Here's the drawing with two shaded views (mm, measured from the low corner). I have some questions. A direction names the side the tool comes from. Round coordinates to 2 decimals unless told otherwise and drop trailing zeros. Loops run counter-clockwise (first coordinate to the right, second up) from the corner with the lowest first, then second, coordinate; pieces in that order, holes last. Notation, with made-up numbers: (46, 34) -> (91, 34) arc R20 ccw to (91, 68) -> close; hole circle Ø11 at (58.25, 61.25). An arc over 180 degrees is marked (long way). Write each question's results on one line, items separated by ' | '.
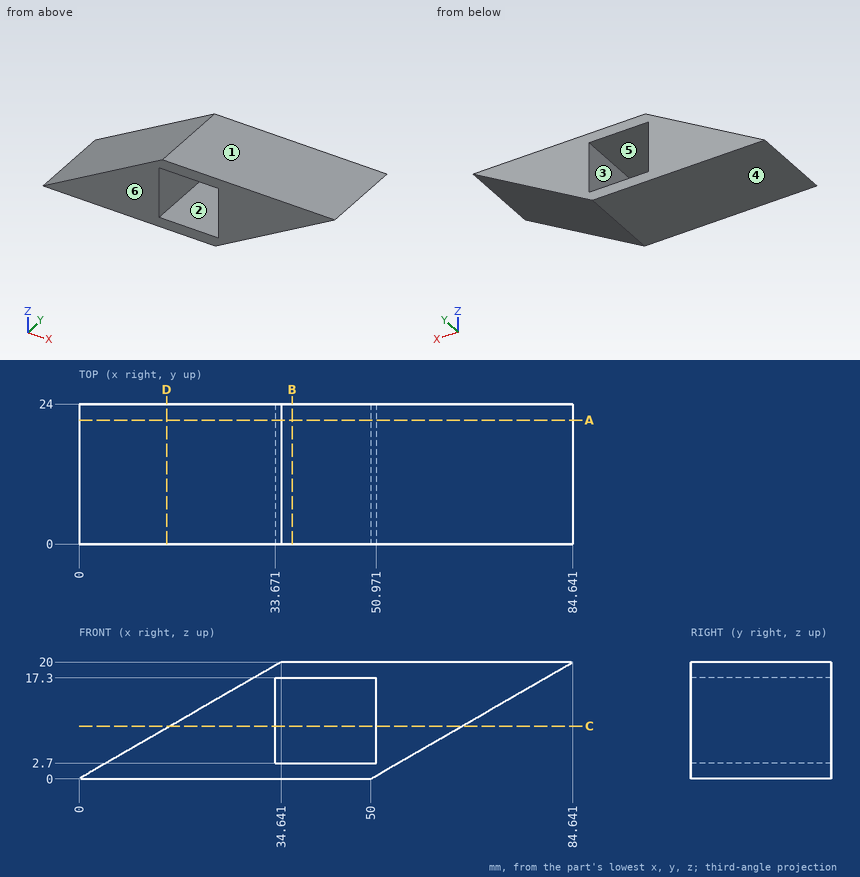
1. Will these pins go through, and if not, where does the flat tip stop? pin 1 (6 mm diameter, centred on y = 11.5, z = 5.5, fed in from +X) (1 decimal); pin 2 (5 mm diameter, centred on x = 25, y = 17, fed in from +Z); pin 3 (11.5 mm diameter, centred on y = 13, z = 12.5, fed in from -X).
Final values:
pin 1: x = 64.7 | pin 2: z = 15.88 | pin 3: x = 11.69
2. Please list where these lines run through material, in increasing order: line 1 (Z direction, x = 44.5, y = 16.25); line 2 (X direction, y = 20, z = 13.25); line 3 (X direction, y = 3, z = 3.75) (1 decimal). Write a range as from..to.
Final values:
line 1: 0..2.7, 17.3..20 | line 2: 22.95..33.67, 50.97..72.95 | line 3: 6.5..33.7, 51..56.5
3. We'd pull the mould along Z, two halves only. Please class the marked faces 3, 4, 5 and 6: pulls with the +Z half, pulls with the -Z half, needs draft (parallel to the pull), parting line crosses it, or undercut.
Final values:
face 3: undercut | face 4: pulls with the -Z half | face 5: undercut | face 6: needs draft
4. If we section it at A-A (y = 21.25): List the corners of the cut face in (x, z) for me.
Final values:
outline: (0, 0) -> (50, 0) -> (84.64, 20) -> (34.64, 20) -> close; hole (33.67, 2.7) -> (50.97, 2.7) -> (50.97, 17.3) -> (33.67, 17.3) -> close
5. If we section it at B-B (x = 36.5): List the corners of the cut face in (y, z) for me.
Final values:
outline: (0, 0) -> (24, 0) -> (24, 2.7) -> (0, 2.7) -> close; (0, 17.3) -> (24, 17.3) -> (24, 20) -> (0, 20) -> close
6. If we section it at C-C (z = 9): List the corners of the cut face in (x, y) for me.
Final values:
outline: (15.59, 0) -> (33.67, 0) -> (33.67, 24) -> (15.59, 24) -> close; (50.97, 0) -> (65.59, 0) -> (65.59, 24) -> (50.97, 24) -> close
7. On a 3-axis mill with a long thin cutter (end or side, diameter ignored), from which of +Z, -Z, +X, -X, +Y, -Y can I reach the whole of each face in a straight line? I mean the marked faces 1 and 2. Say none if no direction works.
Final values:
face 1: +Z, +X, -X, +Y, -Y | face 2: +Y, -Y
8. If we section it at D-D (x = 15): List the corners of the cut face in (y, z) for me.
Final values:
outline: (0, 0) -> (24, 0) -> (24, 8.66) -> (0, 8.66) -> close
